Build history of the part. All positions in model axes, mm. Face numbers are marked on the shaded views. A direction names the side the tool comes from. Coordinates: 2 decimals unless noted, no trailing zeros. Loops run counter-clockwise (first coordinate to the right, second up) from the corner with the lowest first, then second, coordinate; pieces in that order, holes last. Notation, with made-up numbers: (26.25, 6) -> (53.25, 6) arc R17 ccw to (53.25, 15) -> close; hole circle Ø3 at (56.25, -22). An arc over 180 degrees is marked (long way). One line per item, written item: value. Start each with the question number.
```python
from build123d import *

# Parameters (mm, degrees)
F1_DEPTH   = 25.4
F2_W       = 13.9918979257
F2_H       = 6.35
F1_FACE1_W = 26.0131005198
F1_FACE1_H = 25.4
F1_FACE_W  = 13.9918979257
F1_FACE_H  = 25.4
F3_DEPTH   = 25.4


with BuildPart() as f1:
    # F0 (on Top) → F1 (new body)
    with BuildSketch(Plane.XY):
        Polygon((0, 35.8665511012), (0, 0), (53.9968963712, 0), (53.9968963712, 35.8665511012), (40.0049984455, 35.8665511012), (40.0049984455, 13.2036199793), (13.9918979257, 13.2036199793), (13.9918979257, 35.8665511012), align=None)
    extrude(amount=F1_DEPTH)

    # F2 (on face) + F1_face1 (on face) + F1_face (on face) → F3 (join)
    with BuildSketch(Plane(origin=(0, 35.8665511012, 0), x_dir=(-1, 0, 0), z_dir=(0, 1, 0))):
        with Locations((-47.0009474084, 3.175)):
            Rectangle(F2_W, F2_H)
        with Locations((-47.0009474084, 22.225)):
            Rectangle(F2_W, F2_H)
    with BuildSketch(Plane(origin=(26.9984481856, 13.2036199793, 12.7), x_dir=(-1, 0, 0), z_dir=(0, 1, 0))):
        Rectangle(F1_FACE1_W, F1_FACE1_H)
    with BuildSketch(Plane(origin=(47.0009474084, 35.8665511012, 12.7), x_dir=(-1, 0, 0), z_dir=(0, 1, 0))):
        with Locations((40.0049984455, 0)):
            Rectangle(F1_FACE_W, F1_FACE_H)
    extrude(amount=F3_DEPTH)


solid = f1.part
```
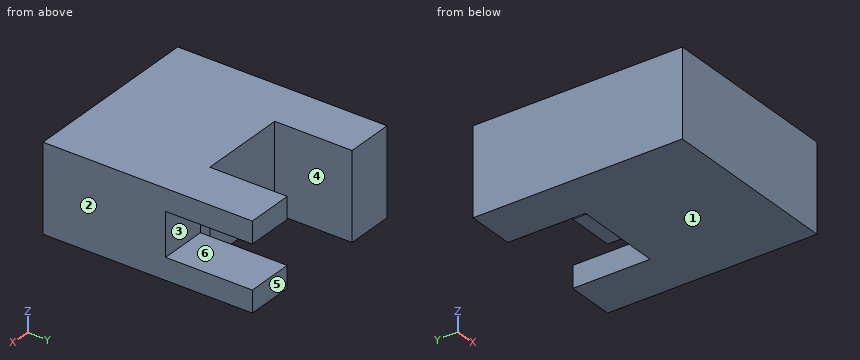
Item 1: Band-saw the part on C-C, the plane z = 4. List the corners of the cut face in (x, y) (3 decimals), and give its area (3 significant figures).
Item 2: Probe probe 1 along Z at (x, y) = (52.5, 37.5); probe 2 along X at (y, z) = (58, 12.25); probe 3 along Y at (x, z) = (28.5, 24). List the from-to ranges inside material, lowest first.
Item 3: Two-plate mould, pull along Z, no slides. Class the marked faces 1, 2 and 3: +Z half, -Z half, draft (parallel to the pull), parting line (faces both ways), or undercut.
Item 4: Band-saw the part on B-B, the plane x = 48. List the corners of the cut face in (y, z), and give its area (3 significant figures).
Item 5: Band-saw the part on D-D, the plane x = 28.5. List the corners of the cut face in (y, z), and give its area (3 significant figures).
Item 6: Band-saw the part on A-A, the plane y = 58. List the corners of the cut face in (x, z) (3 decimals).
Item 7: Drop flat-ended pins along their axis: pin 1 Ø5 at (x, z) = (29.5, 9.5) entering from +Y; pin 2 Ø3 at (y, z) = (37.5, 15) entering from +X (3 decimals); pin 3 Ø4 at (y, z) = (46.5, 14.5) entering from +X. Give the stop position or say it passes through.
Item 8: Tool access for the marked faces 4, 5 and 6: list every direction of +Z, -Z, +X, -X, +Y, -Y with a clear straight run to the whole face (end or side of a thin tool).
Worked out:
1. outline: (0, 0) -> (53.997, 0) -> (53.997, 61.267) -> (40.005, 61.267) -> (40.005, 38.604) -> (13.992, 38.604) -> (13.992, 61.267) -> (0, 61.267) -> close
1. area: 2,720 mm²
2. probe 1: z = 0 to 6.35, 19.05 to 25.4
2. probe 2: x = 0 to 13.99
2. probe 3: y = 0 to 38.6
3. face 1: -Z half
3. face 2: draft
3. face 3: undercut
4. outline: (0, 0) -> (61.27, 0) -> (61.27, 6.35) -> (35.87, 6.35) -> (35.87, 19.05) -> (61.27, 19.05) -> (61.27, 25.4) -> (0, 25.4) -> close
4. area: 1,230 mm²
5. outline: (0, 0) -> (38.6, 0) -> (38.6, 25.4) -> (0, 25.4) -> close
5. area: 981 mm²
6. outline: (0, 0) -> (13.992, 0) -> (13.992, 25.4) -> (0, 25.4) -> close; (40.005, 0) -> (53.997, 0) -> (53.997, 6.35) -> (40.005, 6.35) -> close; (40.005, 19.05) -> (53.997, 19.05) -> (53.997, 25.4) -> (40.005, 25.4) -> close
7. pin 1: stops at y = 38.6
7. pin 2: stops at x = 40.005
7. pin 3: stops at x = 13.99
8. face 4: +Z, -Z, +Y
8. face 5: +Z, -Z, +X, -X, +Y
8. face 6: +X, +Y
